from build123d import *

# Parameters (mm, degrees)
SKETCH_2_R           = 21.5
EXTRUDE_1_DEPTH      = 7
SKETCH_3_R           = 23.5
EXTRUDE_2_DEPTH      = 4
SKETCH_6_R           = 1.25
SKETCH_6_R_2         = 8
CUT_EXTRUDE_1_DEPTH  = 15
SKETCH_9_R           = 14.98
SKETCH_9_R_2         = 14.02
EXTRUDE_3_DEPTH      = 5.5
SKETCH_7_R           = 3.5
CUT_EXTRUDE_3_DEPTH  = 3
SKETCH_10_R          = 1.25
CUT_EXTRUDE_4_DEPTH  = 22
CUT_EXTRUDE_5_DEPTH  = 3
SKETCH_12_R          = 14.02
SKETCH_12_R_2        = 1.5
EXTRUDE_4_DEPTH      = 5.5
CUT_EXTRUDE_START    = -3
SKETCH_13_R          = 14.48
CUT_EXTRUDE_10_DEPTH = 33.507041555


with BuildPart() as part:
    # 草图2 → 凸台-拉伸1 (new body)
    with BuildSketch(Plane(origin=(0, 0, 0), x_dir=(1, 0, 0), z_dir=(0, 1, 0))):
        with Locations(Location((0, 0, 0), (0, 0, 270))):
            Circle(SKETCH_2_R)
    extrude(amount=EXTRUDE_1_DEPTH)

    # 草图3 → 凸台-拉伸2 (add)
    with BuildSketch(Plane(origin=(0, 7, 0), x_dir=(1, 0, 0), z_dir=(0, 1, 0))):
        with Locations(Location((0, 0, 0), (0, 0, 270))):
            Circle(SKETCH_3_R)
    extrude(amount=-EXTRUDE_2_DEPTH)

    # 草图6 → 切除-拉伸1 (cut)
    with BuildSketch(Plane(origin=(0, 7, 0), x_dir=(1, 0, 0), z_dir=(0, 1, 0))):
        with Locations(Location((13.435028843, 13.435028843, 0), (0, 0, 270))):
            Circle(SKETCH_6_R)
        with Locations(Location((13.435028843, -13.435028843, 0), (0, 0, 270))):
            Circle(SKETCH_6_R)
        with Locations(Location((-13.435028843, -13.435028843, 0), (0, 0, 270))):
            Circle(SKETCH_6_R)
        with Locations(Location((-13.435028843, 13.435028843, 0), (0, 0, 270))):
            Circle(SKETCH_6_R)
        with Locations(Location((0, 0, 0), (0, 0, 270))):
            Circle(SKETCH_6_R_2)
    extrude(amount=-CUT_EXTRUDE_1_DEPTH, mode=Mode.SUBTRACT)

    # 草图9 → 凸台-拉伸3 (add)
    with BuildSketch(Plane(origin=(0, 7, 0), x_dir=(1, 0, 0), z_dir=(0, 1, 0))):
        with Locations(Location((0, 0, 0), (0, 0, 270))):
            Circle(SKETCH_9_R)
        with Locations(Location((0, 0, 0), (0, 0, 270))):
            Circle(SKETCH_9_R_2, mode=Mode.SUBTRACT)
    extrude(amount=EXTRUDE_3_DEPTH)

    # 草图7 → 切除-拉伸3 (cut)
    with BuildSketch(Plane(origin=(0, 7, 0), x_dir=(1, 0, 0), z_dir=(0, 1, 0))):
        with Locations(Location((-13.435028843, 13.435028843, 0), (0, 0, 270))):
            Circle(SKETCH_7_R)
        with Locations(Location((13.435028843, 13.435028843, 0), (0, 0, 270))):
            Circle(SKETCH_7_R)
        with Locations(Location((13.435028843, -13.435028843, 0), (0, 0, 270))):
            Circle(SKETCH_7_R)
        with Locations(Location((-13.435028843, -13.435028843, 0), (0, 0, 270))):
            Circle(SKETCH_7_R)
    extrude(amount=-CUT_EXTRUDE_3_DEPTH, mode=Mode.SUBTRACT)

    # 草图10 → 切除-拉伸4 (cut)
    with BuildSketch(Plane(origin=(0, 7, 0), x_dir=(1, 0, 0), z_dir=(0, 1, 0))):
        with Locations(Location((7.778174593, 7.778174593, 0), (0, 0, 270))):
            Circle(SKETCH_10_R)
        with Locations(Location((7.778174593, -7.778174593, 0), (0, 0, 270))):
            Circle(SKETCH_10_R)
        with Locations(Location((-7.778174593, -7.778174593, 0), (0, 0, 270))):
            Circle(SKETCH_10_R)
        with Locations(Location((-7.778174593, 7.778174593, 0), (0, 0, 270))):
            Circle(SKETCH_10_R)
    extrude(amount=-CUT_EXTRUDE_4_DEPTH, mode=Mode.SUBTRACT)

    # 草图11 → 切除-拉伸5 (cut)
    with BuildSketch(Plane.XZ):
        with BuildLine():
            Line((18.619546181, 10.75), (16.887495374, 9.75))
            ThreePointArc((16.887495374, 9.75), (18.835553613, 5.046971379), (19.5, 0))
            Line((19.5, 0), (21.5, 0))
            ThreePointArc((21.5, 0), (20.767405265, 5.56460947), (18.619546181, 10.75))
        make_face()
        with BuildLine():
            Line((0, 21.5), (0, 19.5))
            ThreePointArc((0, 19.5), (5.046971379, 18.835553613), (9.75, 16.887495374))
            Line((9.75, 16.887495374), (10.75, 18.619546181))
            ThreePointArc((10.75, 18.619546181), (5.56460947, 20.767405265), (0, 21.5))
        make_face()
    extrude(amount=-CUT_EXTRUDE_5_DEPTH, mode=Mode.SUBTRACT)

    # 草图12 → 凸台-拉伸4 (add)
    with BuildSketch(Plane(origin=(0, 7, 0), x_dir=(1, 0, 0), z_dir=(0, 1, 0))):
        Circle(SKETCH_12_R)
        with Locations(Location((7.778174593, 7.778174593, 0), (0, 0, 270))):
            Circle(SKETCH_12_R_2, mode=Mode.SUBTRACT)
        with Locations(Location((7.778174593, -7.778174593, 0), (0, 0, 270))):
            Circle(SKETCH_12_R_2, mode=Mode.SUBTRACT)
        with Locations(Location((-7.778174593, -7.778174593, 0), (0, 0, 270))):
            Circle(SKETCH_12_R_2, mode=Mode.SUBTRACT)
        with Locations(Location((-7.778174593, 7.778174593, 0), (0, 0, 270))):
            Circle(SKETCH_12_R_2, mode=Mode.SUBTRACT)
    extrude(amount=EXTRUDE_4_DEPTH)

    # 草图13 → 切除-拉伸10 (cut, through all)
    with BuildSketch(Plane(origin=(0, 12.5, 0), x_dir=(1, 0, 0), z_dir=(0, 1, 0)).offset(CUT_EXTRUDE_START)):
        with Locations(Location((0, 0, 0), (0, 0, 270))):
            Circle(SKETCH_13_R)
    extrude(amount=-CUT_EXTRUDE_10_DEPTH, mode=Mode.SUBTRACT)


solid = part.part
The listing builds one solid part. Answer for the finished solid, in the listing's coordinates (mm). A direction names the side the tool comes from. Give positions to 0.01 mm unless a question says otherwise; leave off trailing zeros. Write each loop counter-clockwise with the first axis right and the second up, starting at its lowest first coordinate (ties: lowest second). Pieces come first, ordered by that corner, then holes. Notation, with made-up numbers: (44, 0) - (54, 0) arc R21 cw to (54, 18) - close; hole circle Ø9 at (14.5, -21.75). An arc over 180 degrees is marked (long way). Use a Markdown table: item, result.
1. Each of these flat-tipped pins is pushed along its axis until it touches: P1, Ø3, axis at x = -9, z = 13, coming from the -Y side; P2, Ø2, axis at x = -13.44, z = 13.44, coming from the +Y side; P3, Ø3.5, axis at x = 13.5, z = 12.5, coming from the +Y side; P4, Ø1, axis at y = 1, z = 20.5, coming from the +X side. Where does it stop, or does it pass through?
Values follow:
| item | result |
|---|---|
| P1 | stops at y = 0 |
| P2 | passes through |
| P3 | stops at y = 4 |
| P4 | stops at x = 0 |
2. For a pull along X with two mould halves and no side action, classify faces 1 (the cylindrical face through (-9.965, 5.521, 12.979)), 2 (the flat face through (0, 1, 21)), 3 (the cylindrical face through (15.88, 5.03, -17.32)) as released by +X, released by -X, zero draft, split by the parting line, or undercut.
Values follow:
| item | result |
|---|---|
| face 1 | undercut |
| face 2 | released by +X |
| face 3 | split by the parting line |
3. A tool of negligible diameter and unlimited length cuts with its end or side. For faces 4 (the flat face through (10.8, 7, -10.8)), 5 (the flat face through (20, 1, 0)), 6 (the flat face through (10.24, 1.48, 17.74)), from which of +Z, -Z, +X, -X, +Y, -Y can it reach the whole face along a straight path? Write none if from no direction.
Values follow:
| item | result |
|---|---|
| face 4 | +Y |
| face 5 | +Z, +X, -Y |
| face 6 | +Z, -Y |
4. Find the intervals of material crossed by probe 1 along X at (y, z) = (4.5, 15.5); probe 2 along Y at (x, z) = (-11.5, -19.5); probe 3 along Y at (x, z) = (-9, 17), in increasing order. Write a range as from..to.
Values follow:
| item | result |
|---|---|
| probe 1 | x = -17.66..-16.26, -10.61..10.61, 16.26..17.66 |
| probe 2 | y = 3..7 |
| probe 3 | y = 0..7 |
5. Section D-D on y = 1 is taken. Write down the section's boundary in (x, z), plus the area to 3 significant figures.
Values follow:
| item | result |
|---|---|
| outline | (0, 19.5) - (0, 21.5) arc R21.5 ccw (long way) to (21.5, 0) - (19.5, 0) arc R19.5 ccw to (16.89, 9.75) - (18.62, 10.75) arc R21.5 ccw to (10.75, 18.62) - (9.75, 16.89) arc R19.5 ccw to start; hole circle Ø2.5 at (-13.44, -13.44); hole circle Ø2.5 at (-13.44, 13.44); hole circle Ø28.96 at (0, 0); hole circle Ø2.5 at (13.44, -13.44); hole circle Ø2.5 at (13.44, 13.44) |
| area | 731 mm² |
6. Section A-A on y = 8 is taken. Write down the section's boundary in (x, z), plus the area to 3 significant figures.
Values follow:
| item | result |
|---|---|
| outline | circle Ø29.96 at (0, 0); hole circle Ø28.96 at (0, 0) |
| area | 46.3 mm² |
7. Section B-B on z = -4 is taken. Write down the section's boundary in (x, y).
Values follow:
| item | result |
|---|---|
| outline | (-23.16, 3) - (-21.12, 3) - (-21.12, 0) - (-13.92, 0) - (-13.92, 9.5) - (13.92, 9.5) - (13.92, 0) - (21.12, 0) - (21.12, 3) - (23.16, 3) - (23.16, 7) - (14.44, 7) - (14.44, 12.5) - (-14.44, 12.5) - (-14.44, 7) - (-23.16, 7) - close |
8. Section C-C on x = -3.5 is taken. Write down the section's boundary in (y, z), plus the area to 3 significant figures.
Values follow:
| item | result |
|---|---|
| outline | (0, -21.21) - (3, -21.21) - (3, -23.24) - (7, -23.24) - (7, -14.57) - (12.5, -14.57) - (12.5, 14.57) - (7, 14.57) - (7, 23.24) - (3, 23.24) - (3, 21.21) - (0, 21.21) - (0, 14.05) - (9.5, 14.05) - (9.5, -14.05) - (0, -14.05) - close |
| area | 206 mm² |
